Input: part model. Units: mm. Frame: model coordinates. A direction names the side the tool comes from. Round coordinates to 2 decimals unless told otherwise and drop trailing zeros. Loops run counter-clockwise (first coordinate to the right, second up) from the corner with the lowest first, then second, coordinate; pieces in that order, holes last. Notation, with made-up numbers: M 69,25 L 85,25 A25 ccw 85,57 Z; hole C 21,41.5 d1. An arc over 180 degrees is marked long. Return JSON: item names as keys, results as strings. Group by question number.
1) Mould query, pull axis X, two halves, no side actions, for faces 5 (the face through (-14.7, 7.1, 12.8)), 6 (the face through (-2.965, 7.098, 18.706)), 7 (the face through (-23, 14, 2)). Classes: +X half, -X half, draft (parallel to the pull), parting line (faces both ways), or undercut.
2) Section D-D (x = -21). Output: boundary loops of the cut face in (y, z).
3) Section B-B (x = -6). Output: boundary loops of the cut face in (y, z).
4) Section C-C (y = 10.5). Count the separate pieces of the cut face and the enclosed holes in it, plus the area to 3 significant figures.
5) Access query for faces 1 (the face through (-34, 7, 5)), 2 (the face through (-2.685, 6.902, -0.596)), 3 (the face through (-40.043, -9.86, 0.651)), 4 (the face through (-4, 7, 5)). Directions: +Z, -Z, +X, -X, +Y, -Y. A direction counts if a zero-diameter tool reaches every point of the face in a straight line with its end or side. Return the directions, or none.
6) Contact query for flat-ended pins moving along their axis: P1, Ø5, axis at x = -38.5, y = -3, coming from the +Z side; P2, Ø8, axis at x = -14, z = 8, coming from the -Y side; P3, Ø6, axis at y = -12, z = 6, coming from the +X side. Output: stop coordinate, or through.
7) Material intervals for line 1 (X direction, y = 3, z = 0); line 2 (Z direction, x = -2, y = 5); line 3 (Z direction, x = -44, y = 7), sorted ascending. Write a range as from..to.
from build123d import *

# Parameters (mm, degrees)
SKETCH1_R           = 5
SKETCH1_R_2         = 2.75
BOSS_EXTRUDE1_DEPTH = 14
BOSS_EXTRUDE2_START = -14
BOSS_EXTRUDE2_DEPTH = 14
SKETCH3_R           = 5
BOSS_EXTRUDE3_DEPTH = 20
FILLET2_R           = 5
BOSS_EXTRUDE4_DEPTH = 14
SKETCH5_R           = 1.9
CUT_EXTRUDE1_DEPTH  = 65.306460705


with BuildPart() as part:
    # Sketch1 → Boss-Extrude1 (new body)
    with BuildSketch(Plane(origin=(0, 0, 0), x_dir=(1, 0, 0), z_dir=(0, 1, 0))):
        with Locations(Location((0, 0, 0), (0, 0, 270))):
            Circle(SKETCH1_R)
        with Locations(Location((0, 0, 0), (0, 0, 270))):
            Circle(SKETCH1_R_2, mode=Mode.SUBTRACT)
    extrude(amount=BOSS_EXTRUDE1_DEPTH)

    # Sketch2 → Boss-Extrude2 (add)
    with BuildSketch(Plane(origin=(0, 14, 0), x_dir=(1, 0, 0), z_dir=(0, 1, 0)).offset(BOSS_EXTRUDE2_START)):
        with BuildLine():
            Line((0, 5), (-50, 5))
            Line((-50, 5), (-50, -5))
            Line((-50, -5), (0, -5))
            ThreePointArc((0, -5), (-5, 0), (0, 5))
        make_face()
    extrude(amount=BOSS_EXTRUDE2_DEPTH)

    # Sketch3 → Boss-Extrude3 (add)
    with BuildSketch(Plane.XZ):
        with Locations(Location((-45, 0, 0), (0, 0, 270))):
            Circle(SKETCH3_R)
    extrude(amount=BOSS_EXTRUDE3_DEPTH)

    # Fillet2
    fillet2_edges = [part.edges().sort_by_distance(p)[0] for p in [
        (-50, 7, -5),
        (-50, 7, 5),
    ]]
    fillet(fillet2_edges, radius=FILLET2_R - 0.0001)  # a hair under: the kernel refuses the full size

    # Sketch4 → Boss-Extrude4 (add)
    with BuildSketch(Plane(origin=(0, 14, 0), x_dir=(1, 0, 0), z_dir=(0, 1, 0))):
        with BuildLine():
            Line((-8.357864376, -5), (0, -13.357864376))
            ThreePointArc((0, -13.357864376), (0, -20.428932188), (-7.071067812, -20.428932188))
            Line((-7.071067812, -20.428932188), (-22.5, -5))
            Line((-22.5, -5), (-8.357864376, -5))
        make_face()
    extrude(amount=-BOSS_EXTRUDE4_DEPTH)

    # Sketch5 → Cut-Extrude1 (cut, through all)
    with BuildSketch(Plane(origin=(0, 14, 0), x_dir=(1, 0, 0), z_dir=(0, 1, 0))):
        with Locations(Location((-3.535533906, -16.893398282, 0), (0, 0, 270))):
            Circle(SKETCH5_R)
    extrude(amount=-CUT_EXTRUDE1_DEPTH, mode=Mode.SUBTRACT)


solid = part.part
Returned:
{
 "1": {"face 5": "-X half", "face 6": "undercut", "face 7": "draft"},
 "2": {"outline": "M 0,-5 L 14,-5 L 14,6.5 L 0,6.5 Z"},
 "3": {"outline": "M 0,-5 L 14,-5 L 14,5 L 0,5 Z; M 0,7.36 L 14,7.36 L 14,21.24 L 0,21.24 Z"},
 "4": {"separate pieces": "1", "enclosed holes": "2", "area": "701 mm^2"},
 "5": {"face 1": "+Z, -X, +Y, -Y", "face 2": "+Y, -Y", "face 3": "-Y", "face 4": "+X, +Y, -Y"},
 "6": {"P1": "stops at z = 3", "P2": "stops at y = 0", "P3": "stops at x = -41"},
 "7": {"line 1": "x = -50..-2.75, 2.75..5", "line 2": "z = -5..-1.89, 1.89..5, 11.36..15.77, 18.01..21.65", "line 3": "z = -5..5"}
}
